Study the drawing (mm; zero at the part's minimum x, y, z) and answer. A direction names the side the tool comes from. Give positions to 0.01 mm unless a question says otherwise; leave off trailing zeros. Write each loop counter-clockwise with the first axis right and the second up, starting at its lowest first coordinate (ties: lowest second). Pieces come first, ordered by that corner, then holes.
1) Straight lines are drawn through the part: probe 1 along X at (y, z) = (3, 18.75); probe 2 along Y at (x, z) = (38.5, 16.5); probe 3 along Z at (x, y) = (16, 24). For each, find the intervals that lie inside material, in ascending order.
2) Find section D-D (z = 22.5). Determine the outline of the cut face in (x, y) (3 decimals), plus the area to 3 significant figures.
3) Find section A-A (y = 16.1). Determine the outline of the cut face in (x, z) (3 decimals), plus the area to 3 significant figures.
4) Given pin 1 Ø6 at (x, y) = (23.5, 22.5) entering from -Z, flat-ended and moving along its own axis, determine where the tip first touches the part or whether it passes through.
5) Find section C-C (x = 4.5). Determine the outline of the cut face in (y, z), plus the area to 3 significant figures.
6) Find section B-B (z = 2.5). Determine the outline of the cut face in (x, y) (3 decimals).
7) Determine the mould class of the marked faces 1, 2, 3 and 4 for opening direction Y: pulls with the +Y half, pulls with the -Y half, needs draft (parallel to the pull), parting line crosses it, or undercut.
8) A tool of negligible diameter and unlimited length cuts with its end or side. For the marked faces 5, 6 and 7, from which of +Z, -Z, +X, -X, +Y, -Y can it reach the whole face along a straight path? Write none if from no direction.
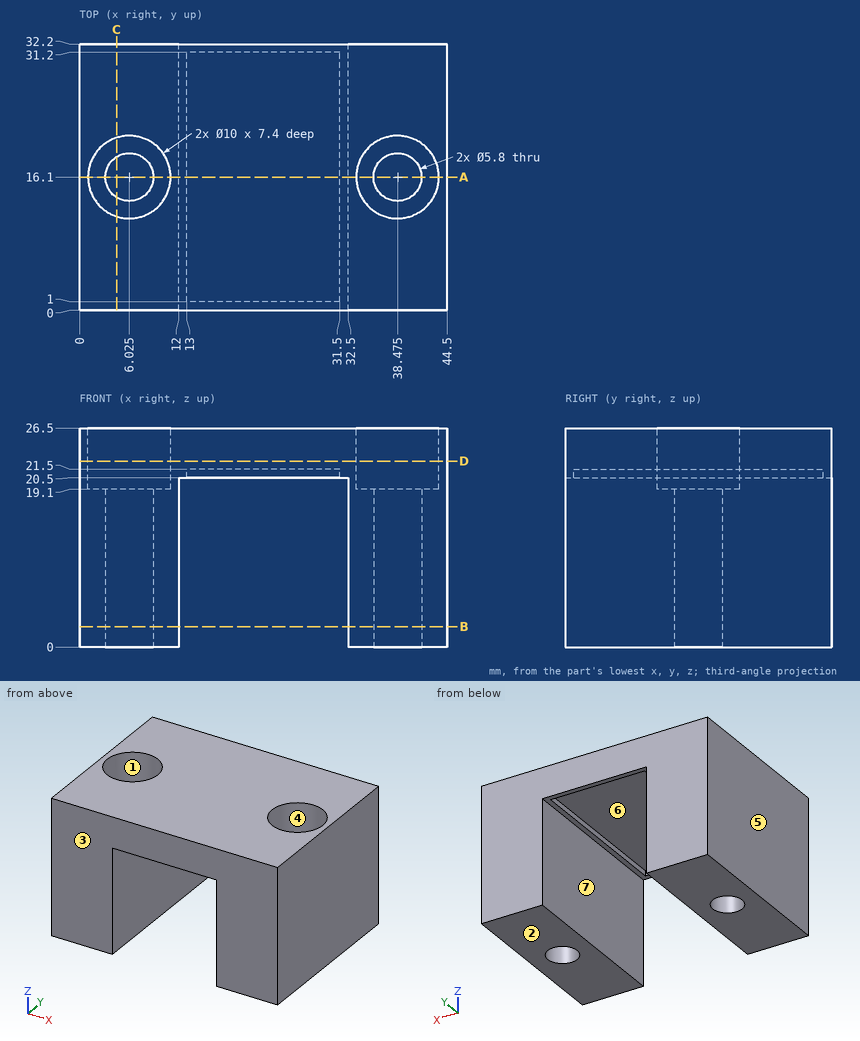
Results:
1. probe 1: x = 0 to 12, 32.5 to 44.5
1. probe 2: y = 0 to 13.2, 19 to 32.2
1. probe 3: z = 21.5 to 26.5
2. outline: (0, 0) - (44.5, 0) - (44.5, 32.2) - (0, 32.2) - close; hole circle Ø10 at (6.025, 16.1); hole circle Ø10 at (38.475, 16.1)
2. area: 1,280 mm2
3. outline: (0, 0) - (3.125, 0) - (3.125, 19.1) - (1.025, 19.1) - (1.025, 26.5) - (0, 26.5) - close; (8.925, 0) - (12, 0) - (12, 20.5) - (13, 20.5) - (13, 21.5) - (31.5, 21.5) - (31.5, 20.5) - (32.5, 20.5) - (32.5, 0) - (35.575, 0) - (35.575, 19.1) - (33.475, 19.1) - (33.475, 26.5) - (11.025, 26.5) - (11.025, 19.1) - (8.925, 19.1) - close; (41.375, 0) - (44.5, 0) - (44.5, 26.5) - (43.475, 26.5) - (43.475, 19.1) - (41.375, 19.1) - close
3. area: 371 mm2
4. pin 1: stops at z = 21.5
5. outline: (0, 0) - (13.63, 0) - (13.63, 19.1) - (11.34, 19.1) - (11.34, 26.5) - (0, 26.5) - close; (18.57, 0) - (32.2, 0) - (32.2, 26.5) - (20.86, 26.5) - (20.86, 19.1) - (18.57, 19.1) - close
5. area: 689 mm2
6. outline: (0, 0) - (12, 0) - (12, 32.2) - (0, 32.2) - close; (32.5, 0) - (44.5, 0) - (44.5, 32.2) - (32.5, 32.2) - close; hole circle Ø5.8 at (6.025, 16.1); hole circle Ø5.8 at (38.475, 16.1)
7. face 1: undercut
7. face 2: needs draft
7. face 3: pulls with the -Y half
7. face 4: undercut
8. face 5: +Z, -Z, -X, +Y, -Y
8. face 6: -Z
8. face 7: -Z, +Y, -Y
